For this review, take the finished solid that the model builds, in its own axes (mm). Face numbers are marked on the shaded views. A direction names the side the tool comes from. Coordinates: 2 decimals unless noted, no trailing zeros. Write each loop counter-clockwise with the first axis right and the second up, starting at its lowest first coordinate (ties: lowest second). Pieces come first, ordered by that corner, then holes. Notation, with made-up numbers: M 9,87.25 L 40,87.25 A9 ccw 40,104.25 Z; hole C 43.5,-18 d4. An arc over 180 degrees is marked long. One line per question, with ' | ' between items.
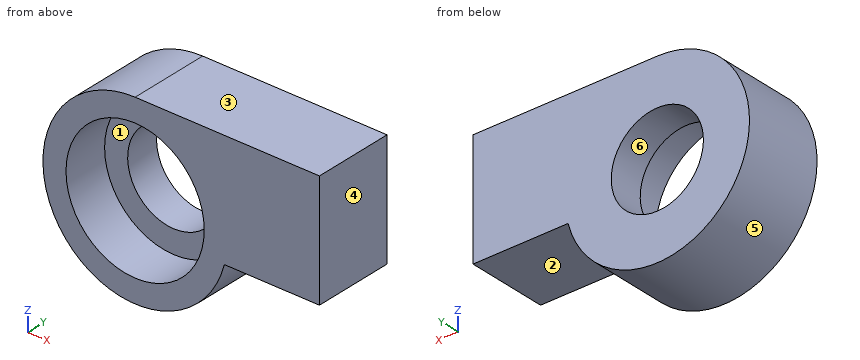
from build123d import *

# Parameters (mm, degrees)
BOSS_EXTRUDE1_DEPTH = 3.5
SKETCH2_R           = 3
CUT_EXTRUDE1_DEPTH  = 2
SKETCH3_R           = 2
CUT_EXTRUDE2_DEPTH  = 10.16515139


with BuildPart() as part:
    # Sketch1 → Boss-Extrude1 (new body)
    with BuildSketch(Plane(origin=(0, 0, 0), x_dir=(1, 0, 0), z_dir=(0, 1, 0))):
        with BuildLine():
            Line((0, -4), (8, -4))
            Line((8, -4), (8, 1))
            Line((8, 1), (3.872983346, 1))
            ThreePointArc((3.872983346, 1), (-3.16227766, 2.449489743), (0, -4))
        make_face()
    extrude(amount=BOSS_EXTRUDE1_DEPTH)

    # Sketch2 → Cut-Extrude1 (cut)
    with BuildSketch(Plane.XZ):
        with Locations(Location((0, 0, 0), (0, 0, 270))):
            Circle(SKETCH2_R)
    extrude(amount=-CUT_EXTRUDE1_DEPTH, mode=Mode.SUBTRACT)

    # Sketch3 → Cut-Extrude2 (cut, through all)
    with BuildSketch(Plane.XZ.offset(-2)):
        with Locations(Location((0, 0, 0), (0, 0, 270))):
            Circle(SKETCH3_R)
    extrude(amount=-CUT_EXTRUDE2_DEPTH, mode=Mode.SUBTRACT)


solid = part.part
1) Machinability: for the marked faces 1, 2 and 3, which of the approach directions +Z, -Z, +X, -X, +Y, -Y give a long, thin tool a straight path to every point of the face, cutting with its end or side? Answer none if there is none.
Responses:
face 1: -Y | face 2: -Z, +X, +Y, -Y | face 3: +Z, +X, -X, +Y, -Y
2) We need section D-D on z = 2.5. State the section outline as (x, y) points.
Responses:
outline: M -3.12,0 L -1.66,0 L -1.66,2 L 1.66,2 L 1.66,0 L 8,0 L 8,3.5 L -3.12,3.5 Z
3) We need section A-A on z = 0. State the section outline as (x, y) points.
Responses:
outline: M -4,0 L -3,0 L -3,2 L -2,2 L -2,3.5 L -4,3.5 Z; M 2,2 L 3,2 L 3,0 L 8,0 L 8,3.5 L 2,3.5 Z
4) We need section B-B on y = 1.5. State the section outline as (x, z) points, then the cut area to 3 significant figures.
Responses:
outline: M 0,4 A4 ccw long 3.87,-1 L 8,-1 L 8,4 Z; hole C 0,0 d6 | area: 45.5 mm^2
5) The part is to be moulded in two halves that separate along Z. For the marked faces 4, 5 and 6, say which applies: +Z half, -Z half, draft (parallel to the pull), parting line (faces both ways), or undercut.
Responses:
face 4: draft | face 5: parting line | face 6: undercut
6) We need section C-C on z = 1.5. State the section outline as (x, y) points, then the cut area to 3 significant figures.
Responses:
outline: M -3.71,0 L -2.6,0 L -2.6,2 L -1.32,2 L -1.32,3.5 L -3.71,3.5 Z; M 1.32,2 L 2.6,2 L 2.6,0 L 8,0 L 8,3.5 L 1.32,3.5 Z | area: 26.6 mm^2
7) To check wall thickness, follow line 1 along X through (y, z) = (2.3, 0); line 2 along Z through (x, y) = (7, 0.55); line 3 along Y through (x, z) = (-0.5, -2.5). State the ranges of each line that lie inside material, in increasing order. Write a range as [from, to].
Responses:
line 1: [-4, -2], [2, 8] | line 2: [-1, 4] | line 3: [2, 3.5]
8) Insertion check: pin 1 Ø1 at (x, y) = (5.5, 1) entering from -Z; pin 2 Ø1.5 at (x, z) = (6.5, -2.5) entering from +Y; pin 3 Ø4 at (x, z) = (-0.5, -0.5) entering from -Y; pin 4 Ø1 at (y, z) = (1, 2) entering from -X. Each pin has a flat end and moves straight along its axis. Give the tip position at first contact, or say it passes through.
Responses:
pin 1: z = -1 | pin 2: through | pin 3: y = 2 | pin 4: x = -3.71
